Check sheet for the modelled part. Datum: model origin and axes. Units: mm. Give positions to 0.01 mm unless a question says otherwise; leave off trailing zeros. Loops run counter-clockwise (first coordinate to the right, second up) from the corner with the lowest first, then second, coordinate; pieces in that order, holes last. Notation, with made-up numbers: (-15, -2) - (10, -2) arc R15 cw to (10, 10) - close; hole circle Ø11 at (7.5, -19.5). An arc over 180 degrees is marked (long way). Use CSV: the item, a comma, the result in double quotes.
from build123d import *

# Parameters (mm, degrees)
ESQUISSE1_W             = 175
ESQUISSE1_H             = 70
ESQUISSE1_W_2           = 100
ESQUISSE1_H_2           = 42
BOSS_EXTRU_1_DEPTH      = 6
ESQUISSE2_R             = 2
ESQUISSE2_W             = 7
ESQUISSE2_H             = 20
ENL_V_MAT_EXTRU_1_DEPTH = 6
ESQUISSE3_R             = 2
ESQUISSE3_R_2           = 6.5
ESQUISSE3_R_3           = 4
ENL_V_MAT_EXTRU_2_DEPTH = 6


with BuildPart() as part:
    # Esquisse1 → Boss.-Extru.1 (new body)
    with BuildSketch(Plane.XY):
        Rectangle(ESQUISSE1_W, ESQUISSE1_H)
        with Locations((-13.5, -2)):
            Rectangle(ESQUISSE1_W_2, ESQUISSE1_H_2, mode=Mode.SUBTRACT)
    extrude(amount=BOSS_EXTRU_1_DEPTH)

    # Esquisse2 → Enlèv. mat.-Extru.1 (cut)
    with BuildSketch(Plane.XY.offset(6)):
        with Locations((-81.5, 19.4)):
            Circle(ESQUISSE2_R)
        with Locations((-81.5, 0)):
            Rectangle(ESQUISSE2_W, ESQUISSE2_H)
    enl_v_mat_extru_1 = extrude(amount=-ENL_V_MAT_EXTRU_1_DEPTH, mode=Mode.SUBTRACT)

    # Symétrie1: Enlèv. mat.-Extru.1 across plane
    add(enl_v_mat_extru_1.mirror(Plane(origin=(0, 0, 0), x_dir=(0, 0, 1), z_dir=(1, 0, 0))), mode=Mode.SUBTRACT)

    # Esquisse3 → Enlèv. mat.-Extru.2 (cut)
    with BuildSketch(Plane.XY.offset(6)):
        with Locations((-73.5, 28)):
            Circle(ESQUISSE3_R)
        with Locations((71, 28)):
            Circle(ESQUISSE3_R)
        with Locations((71, -21.5)):
            Circle(ESQUISSE3_R)
        with Locations((-73.5, -21.5)):
            Circle(ESQUISSE3_R)
        with Locations((59.75, 20)):
            Circle(ESQUISSE3_R_2)
        with Locations((61.25, 1)):
            Circle(ESQUISSE3_R_3)
        with Locations((60.75, -15.25)):
            Circle(ESQUISSE3_R_3)
    extrude(amount=-ENL_V_MAT_EXTRU_2_DEPTH, mode=Mode.SUBTRACT)


solid = part.part
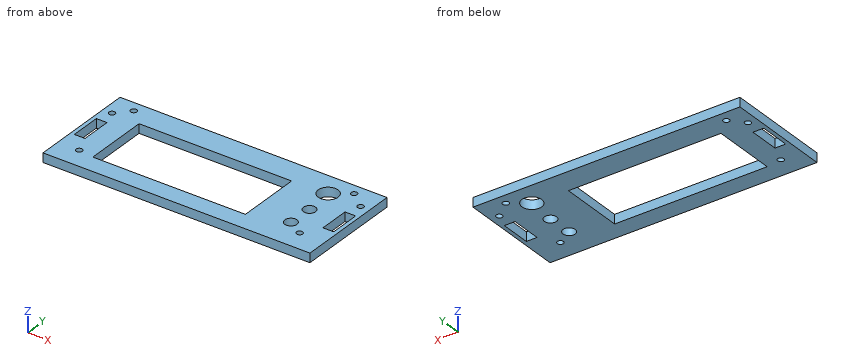
1. Sectioned sample at D-D, the plane y = -15.25. Record the boundary of the cut face in (x, z).
Completed:
outline,"(-87.5, 0) - (-63.5, 0) - (-63.5, 6) - (-87.5, 6) - close; (36.5, 0) - (56.75, 0) - (56.75, 6) - (36.5, 6) - close; (64.75, 0) - (87.5, 0) - (87.5, 6) - (64.75, 6) - close"
2. Sectioned sample at C-C, the plane x = 81.5. Record the boundary of the cut face in (y, z).
Completed:
outline,"(-35, 0) - (-10, 0) - (-10, 6) - (-35, 6) - close; (10, 0) - (17.4, 0) - (17.4, 6) - (10, 6) - close; (21.4, 0) - (35, 0) - (35, 6) - (21.4, 6) - close"
3. Go/stop test with flat-tipped pins: pin 1 Ø10.5 at (x, y) = (60.75, -15.25) entering from -Z; pin 2 Ø2.5 at (x, y) = (-81.5, 19.4) entering from +Z. Record where each tip stops, or that it passes through.
Completed:
pin 1,"stops at z = 0"
pin 2,"passes through"
4. Scan lines: line 1 along Y through (x, z) = (-73.5, 2.4); line 2 along Y through (x, z) = (81.5, 1.6); line 3 along X through (y, z) = (-8.5, 4.15). Record each from-to range of solid material in increasing order.
Completed:
line 1,"y = -35 to -23.5, -19.5 to 26, 30 to 35"
line 2,"y = -35 to -10, 10 to 17.4, 21.4 to 35"
line 3,"x = -87.5 to -85, -78 to -63.5, 36.5 to 78, 85 to 87.5"
5. Sectioned sample at A-A, the plane x = 32. Record the boundary of the cut face in (y, z), and give its area (3 significant figures).
Completed:
outline,"(-35, 0) - (-23, 0) - (-23, 6) - (-35, 6) - close; (19, 0) - (35, 0) - (35, 6) - (19, 6) - close"
area,"168 mm²"
6. Sectioned sample at B-B, the plane y = 1. Record the boundary of the cut face in (x, z).
Completed:
outline,"(-87.5, 0) - (-85, 0) - (-85, 6) - (-87.5, 6) - close; (-78, 0) - (-63.5, 0) - (-63.5, 6) - (-78, 6) - close; (36.5, 0) - (57.25, 0) - (57.25, 6) - (36.5, 6) - close; (65.25, 0) - (78, 0) - (78, 6) - (65.25, 6) - close; (85, 0) - (87.5, 0) - (87.5, 6) - (85, 6) - close"
